Design review of the part built by this model. Coordinates are the model's own, in mm. Face numbers are marked on the shaded views. A direction names the side the tool comes from. Give positions to 0.01 mm unless a question says otherwise; leave off trailing zeros. Loops run counter-clockwise (first coordinate to the right, second up) from the corner with the lowest first, then second, coordinate; pieces in that order, holes last. Notation, with made-up numbers: (40.25, -13.5) -> (46.25, -13.5) arc R23 ccw to (46.25, 15.5) -> close; hole circle Ø5 at (38, -32.5). An arc over 180 degrees is marked (long way). Answer as CSV lines item,"result".
from build123d import *

# Parameters (mm, degrees)
F0_R     = 5
F1_DEPTH = 13
F2_SIZE  = 1
F3_W     = 2
F3_H     = 8
F4_DEPTH = 12.5


with BuildPart() as f1:
    # F0 (on Front) → F1 (new body, symmetric)
    with BuildSketch(Plane.XZ):
        Circle(F0_R)
    extrude(amount=F1_DEPTH, both=True)

    # F2
    f2_edges = [f1.edges().sort_by_distance(p)[0] for p in [
        (-5, -13, 0),
        (-5, 13, 0),
    ]]
    chamfer(f2_edges, length=F2_SIZE)

    # F3 (on Top) → F4 (cut, symmetric)
    with BuildSketch(Plane.XY):
        with Locations((4, 3)):
            Rectangle(F3_W, F3_H)
    extrude(amount=F4_DEPTH, both=True, mode=Mode.SUBTRACT)


solid = f1.part
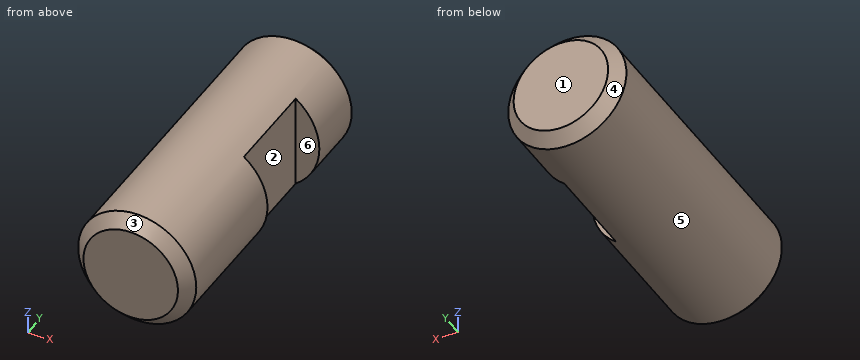
Q1. To check wall thickness, follow probe 1 along X at (y, z) = (10.5, 0.25); probe 2 along Z at (x, y) = (-3, 8.75); probe 3 along X at (y, z) = (-5, -3.5). State the ranges of each line that lie inside material, in increasing order. Write a range as from..to.
Filled sheet:
probe 1,"x = -4.99..4.99"
probe 2,"z = -4..4"
probe 3,"x = -3.57..3.57"
Q2. Clearance check with flat-ended pins moving along their axes: pin 1 Ø1 at (y, z) = (-3.5, -1) entering from +X; pin 2 Ø1.5 at (x, y) = (3.5, -5) entering from -Z; pin 3 Ø1.5 at (x, y) = (-3, -1) entering from +Z. State where each tip first meets the part, or that it passes through.
Filled sheet:
pin 1,"stops at x = 4.97"
pin 2,"stops at z = -4.18"
pin 3,"stops at z = 4.47"
Q3. For the marked faces 1 and 2, list the 3-axis set-ups (+Z, -Z, +X, -X, +Y, -Y) from which the entire face can be reached by the end or side of a thin tool; tool diameter is ignored.
Filled sheet:
face 1,"+Z, -Z, +X, -X, +Y"
face 2,"+Z, -Z, +X"
Q4. We need section B-B, the plane y = -5. State the section outline as (x, z) points, and give its area (3 significant figures).
Filled sheet:
outline,"circle Ø10 at (0, 0)"
area,"78.5 mm^2"
Q5. We need section C-C, the plane y = -0.5. State the section outline as (x, z) points.
Filled sheet:
outline,"(3, -4) -> (3, 4) arc R5 ccw (long way) to start"
Q6. We need section A-A, the plane z = 0. State the section outline as (x, y) points, and give its area (3 significant figures).
Filled sheet:
outline,"(-5, -12) -> (-4, -13) -> (4, -13) -> (5, -12) -> (5, -1) -> (3, -1) -> (3, 7) -> (5, 7) -> (5, 12) -> (4, 13) -> (-4, 13) -> (-5, 12) -> close"
area,"242 mm^2"
Q7. The part is to be moulded in two halves that separate along Y. For the marked faces 3, 4, 5 and 6, say which applies: pulls with the +Y half, pulls with the -Y half, needs draft (parallel to the pull), parting line crosses it, or undercut.
Filled sheet:
face 3,"pulls with the -Y half"
face 4,"pulls with the +Y half"
face 5,"needs draft"
face 6,"undercut"
